from build123d import *

# Parameters (mm, degrees)
F1_DEPTH = 25.4
F2_DEPTH = 2.54


with BuildPart() as f1:
    # F0 (on Top) → F1 (new body)
    with BuildSketch(Plane.XY):
        Polygon((0.34709, 44.238659), (-10.282353, 11.524596), (-41.738984, 14.106456), (-15.933683, -5.868411), (-25.568001, -35.51979), (2.027153, -19.771187), (24.324346, -37.030565), (16.752772, -11.367249), (48.421839, 6.706344), (10.502188, 9.818668), align=None)
        Polygon((-9.564442, 10.446256), (0.300305, 40.806824), (9.724831, 8.863055), (45.068132, 5.962189), (15.550736, -10.883441), (22.460278, -34.302848), (2.112672, -18.552568), (-23.789904, -33.335215), (-14.746518, -5.502534), (-38.409092, 12.813733), align=None, mode=Mode.SUBTRACT)
    extrude(amount=F1_DEPTH)

    # F0 (on Top) → F2 (join)
    with BuildSketch(Plane.XY):
        with BuildLine():
            Line((29.090617, -39.721459), (21.260413, -13.181531))
            Line((21.260413, -13.181531), (53.872965, 5.430511))
            ThreePointArc((53.872965, 5.430511), (55.09367, 8.186757), (52.821757, 10.168026))
            Line((52.821757, 10.168026), (13.417279, 13.40222))
            Line((13.417279, 13.40222), (2.841755, 49.247218))
            ThreePointArc((2.841755, 49.247218), (0.440196, 51.068223), (-2.010111, 49.313362))
            Line((-2.010111, 49.313362), (-12.974523, 15.568374))
            Line((-12.974523, 15.568374), (-45.693581, 18.25385))
            ThreePointArc((-45.693581, 18.25385), (-48.269186, 16.641595), (-47.45611, 13.713795))
            Line((-47.45611, 13.713795), (-20.385559, -7.240452))
            Line((-20.385559, -7.240452), (-30.206309, -37.465611))
            ThreePointArc((-30.206309, -37.465611), (-29.39403, -40.220462), (-26.531641, -40.456542))
            Line((-26.531641, -40.456542), (1.706455, -24.34101))
            Line((1.706455, -24.34101), (25.099682, -42.448785))
            ThreePointArc((25.099682, -42.448785), (28.087545, -42.53731), (29.090617, -39.721459))
        make_face()
        Polygon((-41.738984, 14.106456), (-10.282353, 11.524596), (0.34709, 44.238659), (10.502188, 9.818668), (48.421839, 6.706344), (16.752772, -11.367249), (24.324346, -37.030565), (2.027153, -19.771187), (-25.568001, -35.51979), (-15.933683, -5.868411), align=None, mode=Mode.SUBTRACT)
    extrude(amount=F2_DEPTH)


solid = f1.part
Here's how the part is built. I have some questions about the finished solid (model axes, mm). A direction names the side the tool comes from. Coordinates: 2 decimals unless noted, no trailing zeros. Loops run counter-clockwise (first coordinate to the right, second up) from the corner with the lowest first, then second, coordinate; pieces in that order, holes last.
1. I need wall thicknesses on L1, parallel to X at y = 34, z = 19.25; L2, parallel to X at y = -25, z = 11.25; L3, parallel to Z at x = -22.5, y = -24. Which ranges of each line are inside material? Lowest first, please.
2. For faces 5 (the flat face through (18.957, -22.429, 12.522)), 6 (the flat face through (13.24, -33.27, 1.25)), 7 (the flat face through (-25.8, 12.8, 13.8)), which set-ups out of +Z, -Z, +X, -X, +Y, -Y let a thin tool reach every point of the face, with its end or its side?
3. If we mould it in two halves opening along Y, with no side actions, what happens to faces 1 (the cylindrical face through (55.103, 8.143, 1.252)), 2 (the flat face through (27.149, 7.433, 12.522)), 3 (the flat face through (29.73, 8.24, 13.81)), 4 (the flat face through (-12.61, -32.51, 1.25))? For each: pulls with the +Y half, pulls with the -Y half, needs draft (parallel to the pull), parting line crosses it, or undercut.
4. Imagine slicing it at D-D, the plane x = -22. Please give me the cut outline in (y, z).
5. Imagine slicing it at B-B, the plane x = -35. Please give me the cut outline in (y, z).
6. Imagine slicing it at A-A, the plane z = 19.5. Please give me the cut outline in (x, y), and give its area (3 significant figures).
7. For P1, Ø3, axis at x = -14.5, z = 5, coming from the +Y side; P2, Ø10, axis at y = -29.5, z = 9, coming from the +X side; P3, Ø12, axis at y = -4.5, z = 5, coming from the +X side, each with a flat end and sliding along its axis, tell me the tip position at first contact or that it passes through.
8. Imagine slicing it at C-C, the plane y = -21. Please give me the cut outline in (x, z), and give its area (3 significant figures).
Taken from the geometry:
1. L1: x = -2.98 to -1.91, 2.31 to 3.37
1. L2: x = -22.15 to -21.08, -9.18 to -7.13, 8.78 to 10.44, 19.72 to 20.77
1. L3: z = 0 to 2.54
2. face 5: +Z, -Z
2. face 6: +Z, -Z, -Y
2. face 7: +Z, +Y
3. face 1: parting line crosses it
3. face 2: undercut
3. face 3: pulls with the +Y half
3. face 4: pulls with the -Y half
4. outline: (-37.87, 0) - (-32.31, 0) - (-32.31, 25.4) - (-33.48, 25.4) - (-33.48, 2.54) - (-37.87, 2.54) - close; (-27.83, 0) - (-12.21, 0) - (-12.21, 2.54) - (-24.54, 2.54) - (-24.54, 25.4) - (-27.83, 25.4) - close; (-5.99, 0) - (0.11, 0) - (0.11, 25.4) - (-1.17, 25.4) - (-1.17, 2.54) - (-5.99, 2.54) - close; (11.47, 0) - (16.31, 0) - (16.31, 2.54) - (12.49, 2.54) - (12.49, 25.4) - (11.47, 25.4) - close
5. outline: (4.07, 0) - (10.17, 0) - (10.17, 25.4) - (8.89, 25.4) - (8.89, 2.54) - (4.07, 2.54) - close; (12.53, 0) - (17.38, 0) - (17.38, 2.54) - (13.55, 2.54) - (13.55, 25.4) - (12.53, 25.4) - close
6. outline: (-41.74, 14.11) - (-15.93, -5.87) - (-25.57, -35.52) - (2.03, -19.77) - (24.32, -37.03) - (16.75, -11.37) - (48.42, 6.71) - (10.5, 9.82) - (0.35, 44.24) - (-10.28, 11.52) - close; hole (-38.41, 12.81) - (-14.75, -5.5) - (-23.79, -33.34) - (2.11, -18.55) - (22.46, -34.3) - (15.55, -10.88) - (45.07, 5.96) - (9.72, 8.86) - (0.3, 40.81) - (-9.56, 10.45) - close
6. area: 320 mm2
7. P1: stops at y = 11.99
7. P2: stops at x = 23.58
7. P3: stops at x = 46.06
8. outline: (-24.86, 0) - (-19.78, 0) - (-19.78, 25.4) - (-20.85, 25.4) - (-20.85, 2.54) - (-24.86, 2.54) - close; (-2.18, 0) - (5.27, 0) - (5.27, 25.4) - (3.61, 25.4) - (3.61, 2.54) - (-0.13, 2.54) - (-0.13, 25.4) - (-2.18, 25.4) - close; (18.54, 0) - (23.57, 0) - (23.57, 2.54) - (19.59, 2.54) - (19.59, 25.4) - (18.54, 25.4) - close
8. area: 178 mm2
